Source: CAD feature listing. Evaluate the final solid. Frame: model axes, mm. A direction names the side the tool comes from. Give positions to 0.01 mm unless a question says otherwise; leave off trailing zeros. Order: outer loops, then holes, each group sorted by start corner. A loop starts at its lowest first (then second) coordinate and runs counter-clockwise, first axis right, second up. Notation, with made-up numbers: M 31,25 L 41,25 A20 cw 41,44 Z; hole C -19,45.5 d1. An arc over 180 degrees is marked long. Use CSV: the item, a comma, the result in double quotes. Start each with the question number.
Item 1: Section query B-B on y = 30.5. Count the separate pieces of the cut face and the enclosed holes in it, and give its area (3 significant figures).
Item 2: Section query A-A on z = -14.5. Return loops of the section in (x, y) (3 decimals).
Item 3: Pull-direction query (Y, two-part tool) for faces 1 (the face through (-15.601, -32.375, -6.263)), 2 (the face through (-0.508, -26, -13)); classes: +Y half, -Y half, draft (parallel to the pull), parting line (faces both ways), or undercut.
Item 4: Ray query, probe 1 along Y at (x, z) = (4, -31.5); probe 2 along Y at (x, z) = (18.5, -8); probe 3 along Z at (x, y) = (-34, -8.5). Return the intervals inside material, ascending. Write a range as from..to.
Item 5: Access query for faces 3 (the face through (16.25, -1.67, -17.22)), 4 (the face through (0.508, -26, -13)), 5 (the face through (-15, -23, -15.875)). Directions: +Z, -Z, +X, -X, +Y, -Y. A direction counts if a zero-diameter tool reaches every point of the face in a straight line with its end or side. Return the directions, or none.
Item 6: First-contact query: pin 1 (8.5 mm diameter, centred on x = -17.07, y = 29.56, fed in from -Z); pin 2 (1 mm diameter, centred on y = 22.5, z = -19, fed in from +X); pin 3 (7 mm diameter, centred on x = 0.5, z = -22, fed in from -Y). Flat tips, straight axial feed; report the tip coordinate or a pass-through.
from build123d import *

# Parameters (mm, degrees)
SKETCH3_W           = 1.016
SKETCH3_H           = 40.48125
CUT_EXTRUDE1_DEPTH  = 68.06130649
CUT_EXTRUDE2_REACH  = 69.061
SKETCH4_R           = 3.175
CIRPATTERN1_COUNT   = 3
SKETCH16_W          = 6.35
SKETCH16_H          = 6.35
CUT_EXTRUDE7_DEPTH  = 68.06130649
SKETCH24_R          = 16.335149264
CUT_EXTRUDE13_DEPTH = 68.06130649


# Read off the part's stored shape, not the designer's step: Cut-Extrude3, Cut-Extrude4
with BuildPart() as part:
    # Sketch1 → Revolve1 (revolve)
    with BuildSketch(Plane(origin=(0, 0, 0), x_dir=(0, 0, -1), z_dir=(1, 0, 0)), mode=Mode.PRIVATE) as revolve1_sk:
        Polygon((34.925, -27.1795875), (15.875, -27.7749), (15.875, -26.98115), (12.7, -26.98115), (12.7, -39.97325), (12.192, -40.48125), (0.508, -40.48125), (0, -39.97325), (0, -15.875), (34.925, -15.875), align=None)
    revolve(revolve1_sk.sketch.rotate(Axis((0, 0, 0), (0, 0, -1)), 270), axis=Axis((0, 0, 0), (0, 0, -1)))

    # Sketch3 → Cut-Extrude1 (cut, through all)
    with BuildSketch(Plane.XY):
        with Locations((0, -20.240625)):
            Rectangle(SKETCH3_W, SKETCH3_H)
    extrude(amount=-CUT_EXTRUDE1_DEPTH, mode=Mode.SUBTRACT)

    # Sketch4 → Cut-Extrude2 (cut, up to next)
    with BuildSketch(Plane.XY, mode=Mode.PRIVATE) as cut_extrude2_sk1:
        with Locations((34.13125, 0)):
            Circle(SKETCH4_R)
    cut_extrude2_tool1 = extrude(cut_extrude2_sk1.sketch, amount=-CUT_EXTRUDE2_REACH, mode=Mode.PRIVATE) & part.part
    # Sketch4 → Cut-Extrude2 (cut, up to next)
    with BuildSketch(Plane.XY, mode=Mode.PRIVATE) as cut_extrude2_sk2:
        with Locations((-34.13125, 0)):
            Circle(SKETCH4_R)
    cut_extrude2_tool2 = extrude(cut_extrude2_sk2.sketch, amount=-CUT_EXTRUDE2_REACH, mode=Mode.PRIVATE) & part.part
    cut_extrude2_1 = cut_extrude2_tool1.solids().sort_by_distance((34.13125, 0, 0))[0]
    add(cut_extrude2_1, mode=Mode.SUBTRACT)
    cut_extrude2_2 = cut_extrude2_tool2.solids().sort_by_distance((-34.13125, 0, 0))[0]
    add(cut_extrude2_2, mode=Mode.SUBTRACT)
    cut_extrude2 = cut_extrude2_1 + cut_extrude2_2  # Cut-Extrude2 as one shape, for the pattern or mirror that repeats it

    # Cut-Extrude3 outline → Cut-Extrude3 (revolve, cut)
    with BuildSketch(Plane(origin=(34.13125, 0, 0), x_dir=(1, 0, 0), z_dir=(0, -1, 0))):
        Polygon((3.175, 0), (3.175, -0.137481533), (3.312481533, 0), align=None)
    cut_extrude3 = revolve(axis=Axis((34.13125, 0, 0), (0, 0, 1)), mode=Mode.SUBTRACT)

    # Cut-Extrude4 outline → Cut-Extrude4 (revolve, cut)
    with BuildSketch(Plane(origin=(34.13125, 0, 0), x_dir=(1, 0, 0), z_dir=(0, -1, 0))):
        Polygon((3.312481533, -12.7), (3.175, -12.562518467), (3.175, -12.7), align=None)
    cut_extrude4 = revolve(axis=Axis((34.13125, 0, 0), (0, 0, 1)), mode=Mode.SUBTRACT)

    # CirPattern1: Cut-Extrude2, Cut-Extrude3, Cut-Extrude4 ×3 about axis
    cirpattern1_axis = Axis((0, 0, 0), (0, 0, 1))
    add([cut_extrude2.rotate(cirpattern1_axis, i * 360 / CIRPATTERN1_COUNT) for i in range(1, CIRPATTERN1_COUNT)], mode=Mode.SUBTRACT)
    add([cut_extrude3.rotate(cirpattern1_axis, i * 360 / CIRPATTERN1_COUNT) for i in range(1, CIRPATTERN1_COUNT)], mode=Mode.SUBTRACT)
    add([cut_extrude4.rotate(cirpattern1_axis, i * 360 / CIRPATTERN1_COUNT) for i in range(1, CIRPATTERN1_COUNT)], mode=Mode.SUBTRACT)

    # Sketch16 → Cut-Extrude7 (cut, through all)
    with BuildSketch(Plane.XY):
        with Locations((0, 15.875)):
            Rectangle(SKETCH16_W, SKETCH16_H)
    extrude(amount=-CUT_EXTRUDE7_DEPTH, mode=Mode.SUBTRACT)

    # Sketch24 → Cut-Extrude13 (cut, through all)
    with BuildSketch(Plane.XY):
        Circle(SKETCH24_R)
    extrude(amount=-CUT_EXTRUDE13_DEPTH, mode=Mode.SUBTRACT)


solid = part.part
Verdict:
1,separate pieces,"3"
1,enclosed holes,"0"
1,area,"521 mm2"
2,outline,"M -3.175,16.024 L -3.175,19.05 L 3.175,19.05 L 3.175,16.024 A16.335 cw 0.508,-16.327 L 0.508,-26.976 A26.981 ccw long -0.508,-26.976 L -0.508,-16.327 A16.335 cw Z"
3,face 1,"undercut"
3,face 2,"draft"
4,probe 1,"-26.99..-15.84, 15.84..26.99"
4,probe 2,"-36.01..-32.39, -26.73..26.73, 32.39..36.01"
4,probe 3,"-12.7..0"
5,face 3,"+Z, -Z"
5,face 4,"+Z, -Z, -Y"
5,face 5,"none"
6,pin 1,"z = -12.7"
6,pin 2,"x = 16.79"
6,pin 3,"y = -27.69"
